Check sheet for the modelled part. Datum: model origin and axes. Units: mm. Face numbers are marked on the shaded views. Round coordinates to 2 decimals unless told otherwise and drop trailing zeros.
(1) Mould release check, pull along X, two halves, no side actions. Record for the marked faces 1, 2, 3 and 4: released by +X, released by -X, zero draft, split by the parting line, or undercut.
(2) Thickness scan on probe 1 along X at (y, z) = (39, -1.25); probe 2 along Y at (x, z) = (47.25, 0.75); probe 3 along X at (y, z) = (42.75, 0.75). Record the ranges inside material, lowest first.
(3) Depth check by flat-ended pin: pin 1 (4 mm diameter, centred on x = 48, y = 42, fed in from +Z); pin 2 (1 mm diameter, centred on x = 51, z = 0, fed in from +Y); pin 3 (2 mm diameter, centred on x = 45.5, z = 2, fed in from +Y). Enter the tip coordinate at first touch or a pass-through.
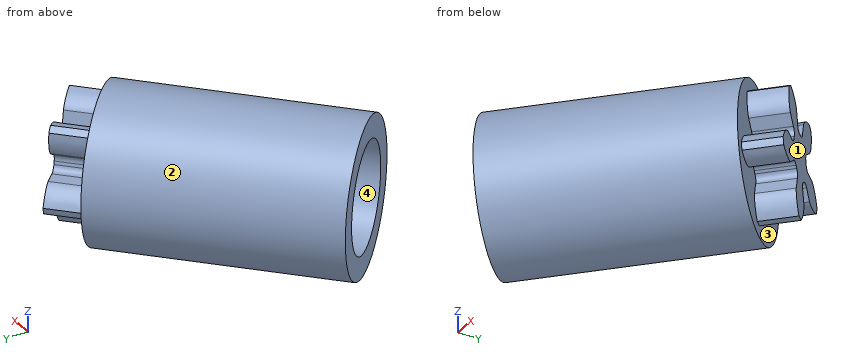
```python
from build123d import *

# Parameters (mm, degrees)
PAD032_DEPTH            = 1.5
SKETCH052_R             = 3
PAD033_DEPTH            = 1.5
SKETCH053_R             = 3
SKETCH053_R_2           = 2.1
PAD034_DEPTH            = 8
BODY020_PITCH_ANGLE     = 90
BODY020_PLACEMENT_ANGLE = 45


with BuildPart() as part:
    # InvoluteGear005 → Pad032 (new body)
    with BuildSketch(Plane.XY):
        with BuildLine():
            Line((1.110631, -0.379257), (1.611002, -0.549274))
            add(Edge.make_bspline(
                [(1.611002, -0.549274), (1.657084, -0.555348), (1.841436, -0.576411), (2.183492, -0.491872), (2.515793, -0.147021)],
                knots=[0, 0, 0, 0, 0, 1, 1, 1, 1, 1], degree=4))
            ThreePointArc((2.515793, -0.147021), (2.520042, 0.0016), (2.515519, 0.150213))
            add(Edge.make_bspline(
                [(2.515519, 0.150213), (2.183492, 0.491872), (1.841436, 0.576411), (1.657084, 0.555348), (1.611002, 0.549274)],
                knots=[0, 0, 0, 0, 0, 1, 1, 1, 1, 1], degree=4))
            Line((1.611002, 0.549274), (1.110631, 0.379257))
            ThreePointArc((1.110631, 0.379257), (0.918725, 0.36265), (0.763436, 0.476619))
            ThreePointArc((0.763436, 0.476619), (0.728115, 0.529007), (0.689206, 0.578787))
            ThreePointArc((0.689206, 0.578787), (0.628802, 0.761694), (0.703899, 0.939076))
            Line((0.703899, 0.939076), (1.020218, 1.362419))
            add(Edge.make_bspline(
                [(1.020218, 1.362419), (1.040234, 1.404369), (1.117234, 1.573189), (1.142534, 1.924628), (0.917248, 2.34723)],
                knots=[0, 0, 0, 0, 0, 1, 1, 1, 1, 1], degree=4))
            ThreePointArc((0.917248, 2.34723), (0.777214, 2.397197), (0.634477, 2.438819))
            add(Edge.make_bspline(
                [(0.634477, 2.438819), (0.206938, 2.228621), (0.020836, 1.92943), (-0.0161, 1.747593), (-0.024564, 1.701889)],
                knots=[0, 0, 0, 0, 0, 1, 1, 1, 1, 1], degree=4))
            Line((-0.024564, 1.701889), (-0.017491, 1.17347))
            ThreePointArc((-0.017491, 1.17347), (-0.060999, 0.985824), (-0.217377, 0.873354))
            ThreePointArc((-0.217377, 0.873354), (-0.278115, 0.855951), (-0.337483, 0.834329))
            ThreePointArc((-0.337483, 0.834329), (-0.530104, 0.833403), (-0.675598, 0.959638))
            Line((-0.675598, 0.959638), (-0.980473, 1.391296))
            add(Edge.make_bspline(
                [(-0.980473, 1.391296), (-1.014184, 1.423295), (-1.150947, 1.548695), (-1.477367, 1.681357), (-1.948903, 1.597689)],
                knots=[0, 0, 0, 0, 0, 1, 1, 1, 1, 1], degree=4))
            ThreePointArc((-1.948903, 1.597689), (-2.039698, 1.479949), (-2.123391, 1.35706))
            add(Edge.make_bspline(
                [(-2.123391, 1.35706), (-2.055597, 0.885492), (-1.828559, 0.616043), (-1.667035, 0.524724), (-1.626183, 0.502551)],
                knots=[0, 0, 0, 0, 0, 1, 1, 1, 1, 1], degree=4))
            Line((-1.626183, 0.502551), (-1.121441, 0.345987))
            ThreePointArc((-1.121441, 0.345987), (-0.956425, 0.246623), (-0.897782, 0.063143))
            ThreePointArc((-0.897782, 0.063143), (-0.9, 0), (-0.897782, -0.063143))
            ThreePointArc((-0.897782, -0.063143), (-0.956425, -0.246623), (-1.121441, -0.345987))
            Line((-1.121441, -0.345987), (-1.626183, -0.502551))
            add(Edge.make_bspline(
                [(-1.626183, -0.502551), (-1.667035, -0.524724), (-1.828559, -0.616043), (-2.055597, -0.885492), (-2.121736, -1.359804)],
                knots=[0, 0, 0, 0, 0, 1, 1, 1, 1, 1], degree=4))
            ThreePointArc((-2.121736, -1.359804), (-2.037816, -1.482538), (-1.946804, -1.60011))
            add(Edge.make_bspline(
                [(-1.946804, -1.60011), (-1.477367, -1.681357), (-1.150947, -1.548695), (-1.014184, -1.423295), (-0.980473, -1.391296)],
                knots=[0, 0, 0, 0, 0, 1, 1, 1, 1, 1], degree=4))
            Line((-0.980473, -1.391296), (-0.675598, -0.959638))
            ThreePointArc((-0.675598, -0.959638), (-0.530104, -0.833403), (-0.337483, -0.834329))
            ThreePointArc((-0.337483, -0.834329), (-0.278115, -0.855951), (-0.217377, -0.873354))
            ThreePointArc((-0.217377, -0.873354), (-0.060999, -0.985824), (-0.017491, -1.17347))
            Line((-0.017491, -1.17347), (-0.024564, -1.701889))
            add(Edge.make_bspline(
                [(-0.024564, -1.701889), (-0.0161, -1.747593), (0.020836, -1.92943), (0.206938, -2.228621), (0.637598, -2.438094)],
                knots=[0, 0, 0, 0, 0, 1, 1, 1, 1, 1], degree=4))
            ThreePointArc((0.637598, -2.438094), (0.780258, -2.396208), (0.9202, -2.345982))
            add(Edge.make_bspline(
                [(0.9202, -2.345982), (1.142534, -1.924628), (1.117234, -1.573189), (1.040234, -1.404369), (1.020218, -1.362419)],
                knots=[0, 0, 0, 0, 0, 1, 1, 1, 1, 1], degree=4))
            Line((1.020218, -1.362419), (0.703899, -0.939076))
            ThreePointArc((0.703899, -0.939076), (0.628802, -0.761694), (0.689206, -0.578787))
            ThreePointArc((0.689206, -0.578787), (0.728115, -0.529007), (0.763436, -0.476619))
            ThreePointArc((0.763436, -0.476619), (0.918725, -0.36265), (1.110631, -0.379257))
        make_face()
    extrude(amount=PAD032_DEPTH)

    # Sketch052 (on Face41 of Pad032) → Pad033 (join)
    with BuildSketch(Plane(origin=(0, 0, 0), x_dir=(1, 0, 0), z_dir=(0, 0, -1))):
        Circle(SKETCH052_R)
    extrude(amount=PAD033_DEPTH)

    # Sketch053 (on Face3 of Pad033) → Pad034 (join)
    with BuildSketch(Plane(origin=(0, 0, -1.5), x_dir=(1, 0, 0), z_dir=(0, 0, -1))):
        Circle(SKETCH053_R)
        Circle(SKETCH053_R_2, mode=Mode.SUBTRACT)
    extrude(amount=PAD034_DEPTH)


with BuildPart() as part_1:
    # Body020 pitch: moved
    add(part.part.rotate(Axis((0, 0, 0), (0, 1, 0)), BODY020_PITCH_ANGLE))


with BuildPart() as part_2:
    # Body020 placement: moved
    add(part_1.part.moved(Location((50, 42.990236, 0))).rotate(Axis((50, 42.990236, 0), (0, 0, 1)), BODY020_PLACEMENT_ANGLE))


solid = part_2.part
```
Derived:
1. face 1: released by +X
1. face 2: split by the parting line
1. face 3: undercut
1. face 4: undercut
2. probe 1: x = 42.15 to 43.62, 48.4 to 49.87
2. probe 2: y = 36.13 to 37.47, 43.01 to 44.35
2. probe 3: x = 45.65 to 46.99, 48.12 to 51.27
3. pin 1: stops at z = 3
3. pin 2: stops at y = 44.61
3. pin 3: stops at y = 43.04
